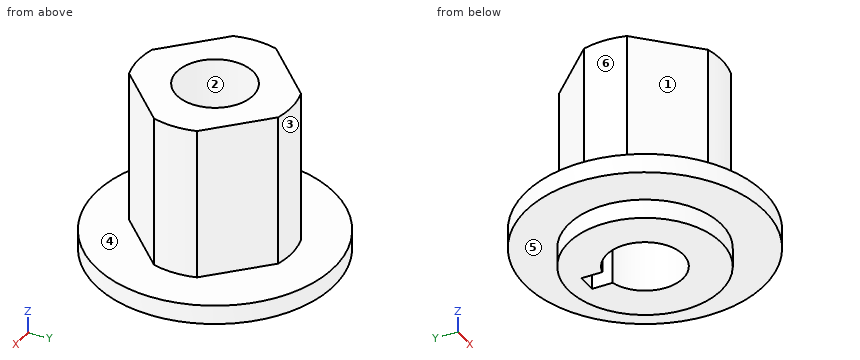
from build123d import *

# Parameters (mm, degrees)
SKETCH1_R           = 12.7
SKETCH1_R_2         = 6.35
BOSS_EXTRUDE1_DEPTH = 3.175
SKETCH2_R           = 19.84375
SKETCH2_R_2         = 6.35
BOSS_EXTRUDE2_DEPTH = 3.175
SKETCH3_R           = 12.7
SKETCH3_R_2         = 6.35
BOSS_EXTRUDE3_DEPTH = 25.4
SKETCH4_W           = 3.175
SKETCH4_H           = 9.525
CUT_EXTRUDE1_DEPTH  = 22.225
SKETCH5_R           = 23.837000359
CUT_EXTRUDE2_DEPTH  = 25.4


with BuildPart() as part:
    # Sketch1 → Boss-Extrude1 (new body)
    with BuildSketch(Plane.XY):
        Circle(SKETCH1_R)
        Circle(SKETCH1_R_2, mode=Mode.SUBTRACT)
    extrude(amount=BOSS_EXTRUDE1_DEPTH)

    # Sketch2 → Boss-Extrude2 (add)
    with BuildSketch(Plane.XY.offset(3.175)):
        Circle(SKETCH2_R)
        Circle(SKETCH2_R_2, mode=Mode.SUBTRACT)
    extrude(amount=BOSS_EXTRUDE2_DEPTH)

    # Sketch3 → Boss-Extrude3 (add)
    with BuildSketch(Plane.XY.offset(6.35)):
        Circle(SKETCH3_R)
        Circle(SKETCH3_R_2, mode=Mode.SUBTRACT)
    extrude(amount=BOSS_EXTRUDE3_DEPTH)

    # Sketch4 → Cut-Extrude1 (cut)
    with BuildSketch(Plane(origin=(0, 0, 0), x_dir=(-1, 0, 0), z_dir=(0, 0, -1))):
        with Locations((0, 4.7625)):
            Rectangle(SKETCH4_W, SKETCH4_H)
    extrude(amount=-CUT_EXTRUDE1_DEPTH, mode=Mode.SUBTRACT)

    # Sketch5 → Cut-Extrude2 (cut)
    with BuildSketch(Plane.XY.offset(31.75)):
        Circle(SKETCH5_R)
        Polygon((0, 15.715448212), (-15.715448212, 0), (0, -15.715448212), (15.715448212, 0), align=None, mode=Mode.SUBTRACT)
    extrude(amount=-CUT_EXTRUDE2_DEPTH, mode=Mode.SUBTRACT)


solid = part.part
The listing builds one solid part. Answer for the finished solid, in the listing's coordinates (mm). Face numbers are marked on the shaded views. A direction names the side the tool comes from. Give positions to 0.01 mm unless a question says otherwise; leave off trailing zeros. Write each loop counter-clockwise with the first axis right and the second up, starting at its lowest first coordinate (ties: lowest second). Pieces come first, ordered by that corner, then holes. Notation, with made-up numbers: (-29, -22.75) -> (-10, -22.75) arc R24 cw to (-10, -5.75) -> close; hole circle Ø10 at (26, 40.5). An arc over 180 degrees is marked (long way). One line per question, with ' | ' between items. Start each with the question number.
1. Section A-A (x = 0) is taken. Determine the outline of the cut face in (y, z) (3 decimals).
2. Given pin 1 Ø1.7 at (y, z) = (7.5, 15) entering from +X; pin 2 Ø10 at (x, z) = (-13, 28.5) entering from -Y; pin 3 Ø1 at (y, z) = (8.5, 16.5) entering from -X; pin 4 Ø2 at (x, y) = (3.5, -0.5) entering from +Z, each flat-ended and moving along its own axis, determine where each tip first touches the part or whether it passes through.
3. Find the intervals of material crossed by probe 1 along Y at (x, z) = (0, 10) (3 decimals); probe 2 along X at (y, z) = (0, 16); probe 3 along Y at (x, z) = (-1, 29), in increasing order.
4. For a pull along Y with two mould halves and no side action, classify the marked faces 1, 2 and 3 as pulls with the +Y half, pulls with the -Y half, needs draft (parallel to the pull), parting line crosses it, or undercut.
5. Section D-D (x = 8.5) is taken. Determine the outline of the cut face in (y, z) (3 decimals), plus the area to 3 significant figures.
6. For the marked faces 4, 5 and 6, determine the directions among +Z, -Z, +X, -X, +Y, -Y from which every point of the face is accessible in a straight line to the end or side of a thin tool.
7. Section B-B (y = 0) is taken. Determine the outline of the cut face in (x, z) (3 decimals).
8. Section C-C (z = 24) is taken. Determine the outline of the cut face in (x, y), plus the area to 3 significant figures.
Response values:
1) outline: (-19.844, 3.175) -> (-12.7, 3.175) -> (-12.7, 0) -> (-6.35, 0) -> (-6.35, 31.75) -> (-12.7, 31.75) -> (-12.7, 6.35) -> (-19.844, 6.35) -> close; (6.35, 22.225) -> (9.525, 22.225) -> (9.525, 0) -> (12.7, 0) -> (12.7, 3.175) -> (19.844, 3.175) -> (19.844, 6.35) -> (12.7, 6.35) -> (12.7, 31.75) -> (6.35, 31.75) -> close
2) pin 1: x = 9.07 | pin 2: y = -7.72 | pin 3: x = -7.72 | pin 4: through
3) probe 1: -12.7 to -6.35, 9.525 to 12.7 | probe 2: -12.7 to -6.35, 6.35 to 12.7 | probe 3: -12.66 to -6.27, 6.27 to 12.66
4) face 1: pulls with the -Y half | face 2: undercut | face 3: pulls with the +Y half
5) outline: (-17.931, 3.175) -> (-9.436, 3.175) -> (-9.436, 0) -> (9.436, 0) -> (9.436, 3.175) -> (17.931, 3.175) -> (17.931, 6.35) -> (7.215, 6.35) -> (7.215, 31.75) -> (-7.215, 31.75) -> (-7.215, 6.35) -> (-17.931, 6.35) -> close | area: 540 mm2
6) face 4: +Z | face 5: -Z | face 6: +Z, -X
7) outline: (-19.844, 3.175) -> (-12.7, 3.175) -> (-12.7, 0) -> (-6.35, 0) -> (-6.35, 31.75) -> (-12.7, 31.75) -> (-12.7, 6.35) -> (-19.844, 6.35) -> close; (6.35, 0) -> (12.7, 0) -> (12.7, 3.175) -> (19.844, 3.175) -> (19.844, 6.35) -> (12.7, 6.35) -> (12.7, 31.75) -> (6.35, 31.75) -> close
8) outline: (-12.21, -3.51) -> (-3.51, -12.21) arc R12.7 ccw to (3.51, -12.21) -> (12.21, -3.51) arc R12.7 ccw to (12.21, 3.51) -> (3.51, 12.21) arc R12.7 ccw to (-3.51, 12.21) -> (-12.21, 3.51) arc R12.7 ccw to start; hole circle Ø12.7 at (0, 0) | area: 327 mm2
